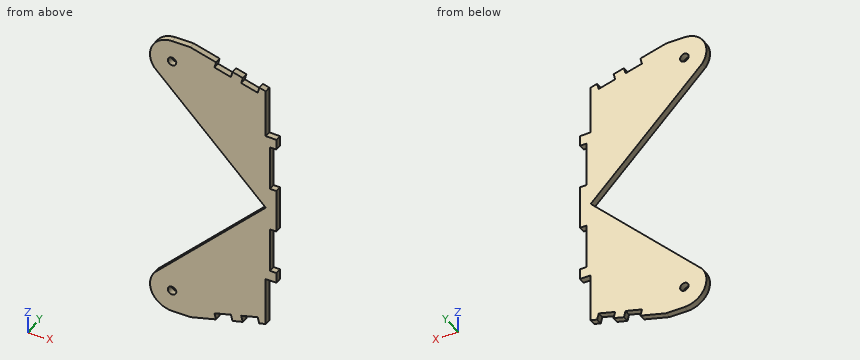
from build123d import *

# Parameters (mm, degrees)
SKETCH1_R           = 3.175
BOSS_EXTRUDE1_DEPTH = 4.7625
SKETCH3_W           = 4.7625
SKETCH3_H           = 33.783
CUT_EXTRUDE2_DEPTH  = 10


with BuildPart() as part:
    # Sketch1 → Boss-Extrude1 (new body)
    with BuildSketch(Plane(origin=(0, 0, 0), x_dir=(1, 0, 0), z_dir=(0, 1, 0))):
        with BuildLine():
            Line((0, 0), (-83.629476528, 83.629476528))
            ThreePointArc((-83.629476528, 83.629476528), (-85.081850373, 100.91197572), (-70.310188895, 110))
            Line((-70.310188895, 110), (-56.601944845, 110))
            Line((-56.601944845, 110), (0, 94.833554589))
            Line((0, 94.833554589), (0, 58.293))
            Line((0, 58.293), (8, 58.293))
            Line((8, 58.293), (8, -58.293))
            Line((8, -58.293), (0, -58.293))
            Line((0, -58.293), (0, -94.833554589))
            Line((0, -94.833554589), (-56.601944845, -110))
            Line((-56.601944845, -110), (-70.310188895, -110))
            ThreePointArc((-70.310188895, -110), (-85.081850373, -100.91197572), (-83.629476528, -83.629476528))
            Line((-83.629476528, -83.629476528), (0, 0))
        make_face()
        with Locations((-70.310188895, 93.451069294)):
            Circle(SKETCH1_R, mode=Mode.SUBTRACT)
        with Locations((-70.310188895, -93.451069294)):
            Circle(SKETCH1_R, mode=Mode.SUBTRACT)
    extrude(amount=BOSS_EXTRUDE1_DEPTH)

    # Sketch3 → Cut-Extrude2 (cut)
    with BuildSketch(Plane(origin=(0, 0, 0), x_dir=(1, 0, 0), z_dir=(0, 1, 0))):
        Polygon((-37.283428319, 104.823619098), (-24.920232031, 101.510910637), (-26.152857733, 96.910688889), (-38.516054022, 100.22339735), align=None)
        Polygon((-17.19282542, 99.440358276), (-4.829629131, 96.127649814), (-6.062254834, 91.527428067), (-18.425451123, 94.840136528), align=None)
        Polygon((-18.425451123, -94.840136528), (-6.062254834, -91.527428067), (-4.829629131, -96.127649814), (-17.19282542, -99.440358276), align=None)
        Polygon((-38.516054022, -100.22339735), (-26.152857733, -96.910688889), (-24.920232031, -101.510910637), (-37.283428319, -104.823619098), align=None)
        with Locations((5.61875, 33.4015)):
            Rectangle(SKETCH3_W, SKETCH3_H)
        with Locations((5.61875, -33.4015)):
            Rectangle(SKETCH3_W, SKETCH3_H)
    extrude(amount=CUT_EXTRUDE2_DEPTH, mode=Mode.SUBTRACT)


solid = part.part
Geometry check sheet. Reference: the model listing, model coordinates, mm. Coordinates: 2 decimals unless noted, no trailing zeros. Order: outer loops, then holes, each group sorted by start corner. A loop starts at its lowest first (then second) coordinate and runs counter-clockwise, first axis right, second up. Notation, with made-up numbers: (46.25, -23.75) -> (53.25, -23.75) arc R17 cw to (53.25, 0.25) -> close; hole circle Ø2 at (-13, 54). An arc over 180 degrees is marked (long way). Use a Markdown table: item, result. Add a question column.
1. Material ranges on L1, parallel to Z at x = 4, y = 3.05; L2, parallel to Z at x = -49, y = 0.6; L3, parallel to Z at x = -66, y = 2, recorded low to high.
2. Cross-section at A-A (x = -41). Enter the section's corners in (y, z).
3. Cross-section at B-B (z = 73.5). Enter the section's corners in (x, y).
4. Cross-section at C-C (x = -10.5). Enter the section's corners in (y, z).
5. Go/stop test with flat-tipped pins: pin 1 Ø1.5 at (x, y) = (-25.5, 0.5) entering from -Z; pin 2 Ø1.4 at (y, z) = (3.5, 80) entering from +X; pin 3 Ø2.5 at (y, z) = (1.5, 41.5) entering from +X; pin 4 Ø5 at (x, z) = (-70.31, -93.45) entering from -Y. Record where each tip stops, or that it passes through.
6. Cross-section at D-D (y = 2.7). Give the number of separate pieces and of enclosed holes in the cut face, and give its area (3 significant figures).
Filled sheet:
| question | item | result |
|---|---|---|
| 1 | L1 | -58.29 to -50.29, -16.51 to 16.51, 50.29 to 58.29 |
| 1 | L2 | -107.96 to -49, 49 to 107.96 |
| 1 | L3 | -110 to -66, 66 to 110 |
| 2 | outline | (0, -105.82) -> (4.76, -105.82) -> (4.76, -41) -> (0, -41) -> close; (0, 41) -> (4.76, 41) -> (4.76, 105.82) -> (0, 105.82) -> close |
| 3 | outline | (-73.5, 0) -> (0, 0) -> (0, 4.76) -> (-73.5, 4.76) -> close |
| 4 | outline | (0, -92.72) -> (4.76, -92.72) -> (4.76, -10.5) -> (0, -10.5) -> close; (0, 10.5) -> (4.76, 10.5) -> (4.76, 92.72) -> (0, 92.72) -> close |
| 5 | pin 1 | z = -101.51 |
| 5 | pin 2 | x = 0 |
| 5 | pin 3 | x = 3.24 |
| 5 | pin 4 | through |
| 6 | separate pieces | 1 |
| 6 | enclosed holes | 2 |
| 6 | area | 10,900 mm2 |
